Part model, mm, in its own coordinate system. A direction names the side the tool comes from. Coordinates: 2 decimals unless noted, no trailing zeros. Loops run counter-clockwise (first coordinate to the right, second up) from the corner with the lowest first, then second, coordinate; pieces in that order, holes last. Notation, with made-up numbers: M -21.75,44.5 L 0.25,44.5 A10 cw 0.25,49.5 Z; hole C 81.5,1.25 d9. An arc over 180 degrees is marked long. Use a Markdown table: item, result. Add a question column.
1) Band-saw the part on A-A (z = -60.5). List the corners of the cut face in (x, y), plus the area to 4 significant figures.
2) Wall check: probe 1 along Y at (x, z) = (-8.5, -22.5); probe 2 along X at (y, z) = (3.5, -92); probe 3 along Y at (x, z) = (-17, -145). Give the ranges that are in metal, low to high. Write a range as from..to.
3) Tool access for faces 1 (the flat face through (-23, 0, 35)), 2 (the flat face through (-5.056, 5.035, -25.323)): list every direction of +Z, -Z, +X, -X, +Y, -Y with a clear straight run to the whole face (end or side of a thin tool).
4) Pin check, flat tips, straight feed: pin 1 Ø6 at (y, z) = (4, -92.5) entering from +X; pin 2 Ø4 at (x, z) = (-7.5, -144.5) entering from +Y; pin 3 Ø5 at (y, z) = (4, 36) entering from -X. Stop position of each tip, or through.
5) Pull direction Y, two halves, no side cores. Call faces 3 (the flat face through (-17.591, 5, 36)), 4 (the cylindrical face through (-22.53, 4.04, 38.07)), 5 (the flat face through (-23, 10, 35)): released by +Y, released by -Y, zero draft, split by the parting line, or undercut.
Autodesk Inventor part; units mm, degrees
ref_plane "Work Plane1" through (0, 7.5, 0) normal (0, 1, 0) x (1, 0, 0)
ref_plane "Work Plane2" through (0, 2.5, 0) normal (0, -1, 0) x (1, 0, 0)
ref_plane "YZ Plane" through (0, 0, 0) normal (1, 0, 0) x (0, 1, 0)
sketch "Sketch1" plane through (0, 0, 0) normal (0, 1, 0) x (-1, 0, 0)
  line L0 (27.5907, 45.377) -> (17.5907, 45.377)
  line L1 (17.5907, 45.377) -> (17.5907, 25.377)
  line L2 (17.5907, 25.377) -> (27.5907, 25.377)
  line L3 (27.5907, 25.377) -> (27.5907, 45.377)
  dimension "d0" = 10
  dimension "d1" = 20
extrude "Extrusion1" add sketch "Sketch1" along normal blind 10
sketch "Sketch2" plane through (-17.5907, 0, 45.377) normal (1, 0, 0) x (0, 0, -1)
  line L0 (0, 10) -> (20, 10) construction
  line L1 (0, 10) -> (10, 10) construction
  line L2 (10, 10) -> (10, 0) construction
  line L3 (10, 0) -> (0, 0) construction
  line L4 (0, 0) -> (0, 10) construction
  line L5 (20, 0) -> (20, 10) construction
  line L6 (0, 10) -> (10, 0) construction
  line L7 (0, 0) -> (20, 0) construction
  line L8 (10, 10) -> (0, 0) construction
  circle A0 centre (5, 5) radius 2.5
  point P0 (45.377, 0)
  dimension "d4" = 5
extrude "Extrusion2" cut sketch "Sketch2" against normal through all
fillet "Fillet1" radius 0.5 2 edges at (-17.5907, 5, 42.877) (-27.5907, 5, 42.877)
fillet "Fillet2" radius 3 2 edges at (-22.5907, 10, 45.377) (-22.5907, 0, 45.377)
ref_plane "Work Plane1" through (0, 7.5, 0) normal (0, 1, 0) x (1, 0, 0)
ref_plane "Work Plane2" through (0, 2.5, 0) normal (0, -1, 0) x (1, 0, 0)
sketch "Sketch7" plane through (0, 7.5, 0) normal (0, 1, 0) x (1, 0, 0)
  line L0 (-32.5907, -25.377) -> (-2.5907, -25.377)
  line L1 (-2.5907, -25.377) -> (-2.5907, 74.623)
  line L2 (-2.5907, 74.623) -> (-32.5907, 74.623)
  line L3 (-32.5907, 74.623) -> (-32.5907, -25.377)
  line L4 (-17.5907, -25.377) -> (-27.5907, -25.377)
  line L5 (-27.5907, -25.377) -> (-27.5907, -42.377)
  line L6 (-17.5907, -42.377) -> (-17.5907, -25.377)
  point P0 (0, 0)
  dimension "d30" = 0
  dimension "d31" = 5
  dimension "d32" = 15
  dimension "d33" = 100
sketch "Sketch8" plane through (0, 2.5, 0) normal (0, -1, 0) x (1, 0, 0)
  line L0 (-42.5907, 25.377) -> (-7.5907, 25.377)
  line L1 (-7.5907, 25.377) -> (-7.5907, -74.623)
  line L2 (-7.5907, -74.623) -> (-42.5907, -74.623)
  line L3 (-42.5907, -74.623) -> (-42.5907, 25.377)
  line L4 (-17.5907, 25.377) -> (-27.5907, 25.377)
  line L5 (-27.5907, 25.377) -> (-27.5907, 42.377)
  line L6 (-17.5907, 42.377) -> (-17.5907, 25.377)
  point P0 (0, 0)
  dimension "d34" = 0
  dimension "d35" = 15
  dimension "d36" = 10
  dimension "d37" = 100
loft "Loft4" add profiles "Sketch8", "Sketch7"
sketch "Sketch9" plane through (-17.5907, 0, 42.377) normal (1, 0, 0) x (0, 0, -1)
  line L0 (17, 7.5) -> (17, 10)
  line L1 (17, 7.5) -> (12, 7.5)
  line L2 (12, 7.5) -> (12, 2.5)
  line L3 (12, 2.5) -> (17, 2.5)
  line L4 (17, 2.5) -> (17, 7.5)
  line L5 (17, 0) -> (17, 2.5)
  point P0 (42.377, 0)
  dimension "d42" = 5
sketch "Sketch10" plane through (-27.5907, 0, 25.377) normal (-1, 0, 0) x (0, 0, 1)
  line L0 (0, 2.5) -> (0, 7.5)
  line L1 (0, 7.5) -> (5, 7.5)
  line L2 (5, 7.5) -> (5, 2.5)
  line L3 (5, 2.5) -> (0, 2.5)
  line L4 (0, 2.5) -> (0, 7.5)
  point P0 (-25.377, 0)
  dimension "d43" = 5
extrude "Extrusion3" add sketch "Sketch10" along normal blind 5
extrude "Extrusion4" add sketch "Sketch9" along normal blind 5
chamfer "Chamfer1" distance 5 angle 45 2 edges at (-12.5907, 5, 30.377) (-32.5907, 5, 30.377)
sketch "Sketch11" plane through (-32.5907, 7.5, -74.623) normal (0, 1, 0) x (1, 0, 0)
  line L0 (30, 0) -> (0, 0)
  line L1 (30, 0) -> (56.7949, 100)
  line L2 (56.7949, 100) -> (26.7949, 100)
  line L3 (26.7949, 100) -> (0, 0)
  line L4 (30, -100) -> (30, 0)
  point P0 (32.5907, -74.623)
  dimension "d52" = 15
  dimension "d53" = 100
sketch "Sketch12" plane through (-42.5907, 2.5, -74.623) normal (0, -1, 0) x (1, 0, 0)
  line L0 (35, 0) -> (0, 0)
  line L1 (0, 0) -> (26.7949, -100)
  line L2 (26.7949, -100) -> (61.7949, -100)
  line L3 (61.7949, -100) -> (35, 0)
  line L4 (0, 0) -> (0, 100)
  point P0 (42.5907, 74.623)
  dimension "d54" = 100
  dimension "d55" = 15
loft "Loft5" add profiles "Sketch11", "Sketch12"
chamfer "Chamfer2" distance 2.5 angle 45 2 edges at (-22.5907, 0, 25.377) (-22.5907, 10, 25.377)
chamfer "Chamfer3" distance 2.5 angle 45 1 edges at (9.2042, 7.5, -174.623)
equation "\"d35\" = d32"
equation "\"d37\" = d33"
equation "\"d43\" = d42"
equation "\"d54\" = d53"
equation "\"d55\" = d52"
properties part number "Gyrocopter Blade"
Entries:
| question | item | result |
|---|---|---|
| 1 | outline | M -42.59,2.5 L -7.59,2.5 L -2.59,7.5 L -32.59,7.5 Z |
| 1 | area | 162.5 mm2 |
| 2 | probe 1 | 2.5..7.5 |
| 2 | probe 2 | -35.93..-1.93 |
| 2 | probe 3 | 2.5..5.87 |
| 3 | face 1 | +Z, -Z, +X, -X, -Y |
| 3 | face 2 | +Z, +X, -Y |
| 4 | pin 1 | x = 1.81 |
| 4 | pin 2 | y = 7.5 |
| 4 | pin 3 | x = -27.59 |
| 5 | face 3 | zero draft |
| 5 | face 4 | undercut |
| 5 | face 5 | released by +Y |
